from build123d import *

# Parameters (mm, degrees)
F1_DEPTH = 3


with BuildPart() as f1:
    # F0 (on Front) → F1 (new body)
    with BuildSketch(Plane.XZ):
        with BuildLine():
            Line((190.392517, 16.33272), (530, 0))
            Line((530, 0), (530, 1683.898172))
            ThreePointArc((530, 1683.898172), (474.778273, 1821.880967), (339.607483, 1883.66728))
            Line((339.607483, 1883.66728), (0, 1900))
            Line((0, 1900), (0, 216.101828))
            ThreePointArc((0, 216.101828), (55.221727, 78.119033), (190.392517, 16.33272))
        make_face()
    extrude(amount=F1_DEPTH)


solid = f1.part
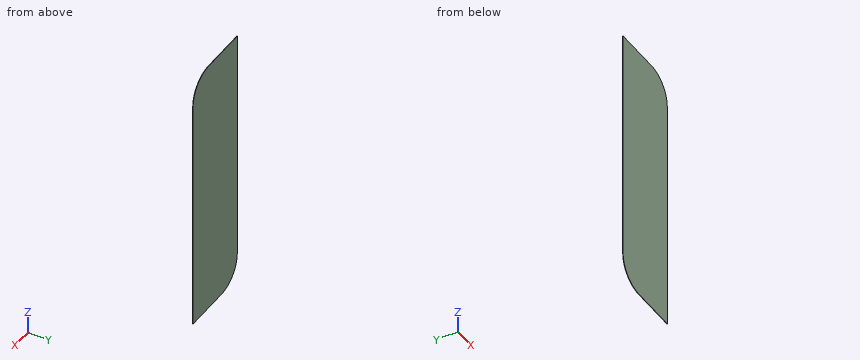
Can you work these out from the model? Positions are in its coordinate system, mm. Coordinates: 2 decimals unless noted, no trailing zeros. Loops run counter-clockwise (first coordinate to the right, second up) from the corner with the lowest first, then second, coordinate; pieces in that order, holes last. Notation, with made-up numbers: M 72.25,6.5 L 108.25,6.5 A15 cw 108.25,14.5 Z; hole C 12,-30 d6. An arc over 180 degrees is marked long. Return JSON: item names as keys, results as strings. Group by question number.
Item 1: I'm going to push a flat-ended pin straight in: pin 1 Ø1 at (x, y) = (366.5, -0.5) entering from -Z. Where does the tip first touch, or does it pass through?
Item 2: Imagine slicing it at B-B (x = 420). Please give me the cut outline in (y, z), and give its area (3 significant figures).
Item 3: Imagine slicing it at A-A (y = -0.8). Please give me the cut outline in (x, z).
Item 4: Imagine slicing it at C-C (x = 54). Please give me the cut outline in (y, z).
Item 5: If I drill on L1, parallel to Z at x = 404, y = -2; L2, parallel to Z at x = 438, y = -0.3; L3, parallel to X at y = -2.5, z = 121.5, over which ranges is the centre line in solid material (lowest first)? Write a range as from..to.
Verdict:
{
 "1": {"pin 1": "stops at z = 7.84"},
 "2": {"outline": "M -3,5.29 L 0,5.29 L 0,1862.5 L -3,1862.5 Z", "area": "5,570 mm^2"},
 "3": {"outline": "M 0,216.1 A200 ccw 190.39,16.33 L 530,0 L 530,1683.9 A200 ccw 339.61,1883.67 L 0,1900 Z"},
 "4": {"outline": "M -3,79.41 L 0,79.41 L 0,1897.4 L -3,1897.4 Z"},
 "5": {"L1": "z = 6.06..1869.7", "L2": "z = 4.42..1852.23", "L3": "x = 23.79..530"}
}
